```python
from build123d import *

# Parameters (mm, degrees)
SKETCH1_R           = 2.25
BOSS_EXTRUDE1_DEPTH = 5
SKETCH2_W           = 7
SKETCH2_H           = 9
BOSS_EXTRUDE2_DEPTH = 20
SKETCH4_W           = 9
SKETCH4_H           = 9
BOSS_EXTRUDE4_DEPTH = 50
SKETCH5_R           = 2.5
CUT_EXTRUDE1_DEPTH  = 25
FILLET1_R           = 5
FILLET2_R           = 5


with BuildPart() as part:
    # Sketch1 → Boss-Extrude1 (new body)
    with BuildSketch(Plane.XY):
        with BuildLine():
            ThreePointArc((4.5, 10), (0, 14.5), (-4.5, 10))
            Line((-4.5, 10), (-4.5, -10))
            ThreePointArc((-4.5, -10), (0, -14.5), (4.5, -10))
            Line((4.5, -10), (4.5, 10))
        make_face()
        with Locations((0, 10)):
            Circle(SKETCH1_R, mode=Mode.SUBTRACT)
        with Locations((0, -10)):
            Circle(SKETCH1_R, mode=Mode.SUBTRACT)
    extrude(amount=BOSS_EXTRUDE1_DEPTH)

    # Sketch2 → Boss-Extrude2 (add)
    with BuildSketch(Plane.XY.offset(5)):
        Rectangle(SKETCH2_W, SKETCH2_H)
    extrude(amount=BOSS_EXTRUDE2_DEPTH)

    # Sketch4 → Boss-Extrude4 (add)
    with BuildSketch(Plane(origin=(3.5, 0, 0), x_dir=(0, 0, -1), z_dir=(1, 0, 0))):
        with Locations((-20.5, 0)):
            Rectangle(SKETCH4_W, SKETCH4_H)
    extrude(amount=BOSS_EXTRUDE4_DEPTH)

    # Sketch5 → Cut-Extrude1 (cut)
    with BuildSketch(Plane(origin=(53.5, 0, 0), x_dir=(0, 0, -1), z_dir=(1, 0, 0))):
        with Locations((-20.5, 0)):
            Circle(SKETCH5_R)
    extrude(amount=-CUT_EXTRUDE1_DEPTH, mode=Mode.SUBTRACT)

    # Fillet1
    fillet1_edges = [part.edges().sort_by_distance(p)[0] for p in [
        (3.5, 0, 16),
    ]]
    fillet(fillet1_edges, radius=FILLET1_R)

    # Fillet2
    fillet2_edges = [part.edges().sort_by_distance(p)[0] for p in [
        (-3.5, 0, 25),
    ]]
    fillet(fillet2_edges, radius=FILLET2_R)


solid = part.part
```
Geometry: final body of the model. Coordinates: model frame, mm. A direction names the side the tool comes from. Give positions to 0.01 mm unless a question says otherwise; leave off trailing zeros. Order: outer loops, then holes, each group sorted by start corner. A loop starts at its lowest first (then second) coordinate and runs counter-clockwise, first axis right, second up. Notation, with made-up numbers: M -5.75,59.5 L 21.25,59.5 A5 cw 21.25,66.5 Z; hole C -19.75,33.5 d4. An arc over 180 degrees is marked long. Answer as CSV lines item,"result". Start each with the question number.
1) Line query: line 1 (Y direction, x = 0, z = 1.55); line 2 (Z direction, x = 50.5, y = -1.5); line 3 (Z direction, x = 51.5, y = 1.75). Output: solid intervals per line, ascending. Write a range as from..to.
2) Set-up query: faces 1 (the cylindrical face through (41, 0, 23)), 2 (the flat face through (31, 0, 16)), 3 (the flat face through (18, -4.5, 20)), 4 (the flat face through (3.5, 0, 8)). Return all of +Z, -Z, +X, -X, +Y, -Y with unobstructed straight access to the full face (end or side cutting, diameter ignored); none if empty.
3) Mould query, pull axis Z, two halves, no side actions, for faces 5 (the cylindrical face through (-2, 0.06, 23.57)), 6 (the flat face through (28.5, 0, 21)), 7 (the flat face through (0, 0, 0)), 8 (the flat face through (-3.5, 0, 12)). Classes: +Z half, -Z half, draft (parallel to the pull), parting line (faces both ways), or undercut.
4) Cut plane A-A (x = 34.5). Output: boundary loops of the cut face in (y, z), then the cut area to 3 significant figures.
5) Cut plane C-C (y = 10.75). Output: boundary loops of the cut face in (x, z).
6) First-contact query: P1, Ø2.5, axis at y = -0.5, z = 20.5, coming from the +X side; P2, Ø4, axis at x = 15.5, z = 22, coming from the +Y side; P3, Ø1.8, axis at y = -1.5, z = 7, coming from the +X side; P4, Ø1.5, axis at x = 15.5, y = 6, coming from the -Z side. Flat tips, straight axial feed; report the tip coordinate or a pass-through.
7) Cut plane B-B (y = 3.5). Output: boundary loops of the cut face in (x, z).
8) Cut plane D-D (z = 21.5). Output: boundary loops of the cut face in (x, y).
Findings below:
1,line 1,"y = -14.5..-12.25, -7.75..7.75, 12.25..14.5"
1,line 2,"z = 16..18.5, 22.5..25"
1,line 3,"z = 16..18.71, 22.29..25"
2,face 1,"+X"
2,face 2,"-Z, +X, +Y, -Y"
2,face 3,"+Z, +X, -X, -Y"
2,face 4,"+X, +Y, -Y"
3,face 5,"+Z half"
3,face 6,"undercut"
3,face 7,"-Z half"
3,face 8,"draft"
4,outline,"M -4.5,16 L 4.5,16 L 4.5,25 L -4.5,25 Z; hole C 0,20.5 d5"
4,area,"61.4 mm²"
5,outline,"M -4.44,0 L -2.12,0 L -2.12,5 L -4.44,5 Z; M 2.12,0 L 4.44,0 L 4.44,5 L 2.12,5 Z"
6,P1,"stops at x = 28.5"
6,P2,"stops at y = 4.5"
6,P3,"stops at x = 3.5"
6,P4,"passes through"
7,outline,"M -4.5,0 L 4.5,0 L 4.5,5 L 3.5,5 L 3.5,11 A5 cw 8.5,16 L 53.5,16 L 53.5,25 L 1.5,25 A5 ccw -3.5,20 L -3.5,5 L -4.5,5 Z"
8,outline,"M -3.27,-4.5 L 53.5,-4.5 L 53.5,-2.29 L 28.5,-2.29 L 28.5,2.29 L 53.5,2.29 L 53.5,4.5 L -3.27,4.5 Z"
